Autodesk Inventor part; units mm, degrees
ref_plane "YZ Plane" through (0, 0, 0) normal (1, 0, 0) x (0, 1, 0)
ref_plane "XZ Plane" through (0, 0, 0) normal (0, 1, 0) x (-1, 0, 0)
ref_plane "XY Plane" through (0, 0, 0) normal (0, 0, 1) x (1, 0, 0)
sketch "Sketch1" plane through (0, 0, 0) normal (0, 0, 1) x (1, 0, 0)
  circle A0 centre (0, 0) radius 11
  circle A1 centre (-15.5, 15.5) radius 1.5
  circle A2 centre (15.5, 15.5) radius 1.5
  circle A3 centre (-15.5, -15.5) radius 1.5
  circle A4 centre (15.5, -15.5) radius 1.5
  line L0 (21.05, -21.05) -> (-21.05, -21.05)
  line L1 (21.05, 21.05) -> (21.05, -21.05)
  line L2 (-21.05, 21.05) -> (21.05, 21.05)
  line L3 (-21.05, -21.05) -> (-21.05, 21.05)
  point P0 (0, 0)
extrude "Extrusion1" add sketch "Sketch1" along normal blind 8
sketch "Sketch2" plane through (-21.05, 21.05, 0) normal (0, 1, 0) x (1, 0, 0)
  line L0 (42.1, 0) -> (0, 0)
  line L1 (0, 0) -> (0, -8)
  line L2 (42.1, -8) -> (0, -8)
  line L3 (42.1, 0) -> (42.1, -8)
  point P0 (21.05, 0)
extrude "Extrusion2" add sketch "Sketch2" along normal blind 50
properties part number "nema17 x plate"
Work out the finished part from the listing and answer in its coordinate system (mm). Round coordinates to 2 decimals unless told otherwise and drop trailing zeros. Write each loop counter-clockwise with the first axis right and the second up, starting at its lowest first coordinate (ties: lowest second). Pieces come first, ordered by that corner, then holes. Notation, with made-up numbers: (-13, -16.5) - (43, -16.5) arc R27 cw to (43, 0.5) - close; hole circle Ø2 at (-8, -3). An arc over 180 degrees is marked (long way). Return JSON: item names as keys, results as strings. Group by question number.
Q1. The part is cut by section C-C on y = 15.5. Write down the section's boundary in (x, z).
Q2. The mould has two halves that part along X. Classify faces 1 (the cylindrical face through (-17, 15.43, 3.94)), 2 (the flat face through (0, 71.05, 4)), 3 (the flat face through (21.05, 26, 4)), 4 (the cylindrical face through (-17, -15.57, 3.94)): released by +X, released by -X, zero draft, split by the parting line, or undercut.
Q3. The part is cut by section B-B on x = 0. Write down the section's boundary in (y, z), then the cut area to 3 significant figures.
Q4. The part is cut by section D-D on x = 15.5. Write down the section's boundary in (y, z).
Q5. Find the intervals of material crossed by L1, parallel to X at y = 14.5, z = 7.5; L2, parallel to Y at x = -15, z = 3.5; L3, parallel to Y at x = 2, z = 3.75, in increasing order.
Q6. The part is cut by section A-A on y = 0. Write down the section's boundary in (x, z).
Solved:
{
 "1": {"outline": "(-21.05, 0) - (-17, 0) - (-17, 8) - (-21.05, 8) - close; (-14, 0) - (14, 0) - (14, 8) - (-14, 8) - close; (17, 0) - (21.05, 0) - (21.05, 8) - (17, 8) - close"},
 "2": {"face 1": "undercut", "face 2": "zero draft", "face 3": "released by +X", "face 4": "undercut"},
 "3": {"outline": "(-21.05, 0) - (-11, 0) - (-11, 8) - (-21.05, 8) - close; (11, 0) - (71.05, 0) - (71.05, 8) - (11, 8) - close", "area": "561 mm²"},
 "4": {"outline": "(-21.05, 0) - (-17, 0) - (-17, 8) - (-21.05, 8) - close; (-14, 0) - (14, 0) - (14, 8) - (-14, 8) - close; (17, 0) - (71.05, 0) - (71.05, 8) - (17, 8) - close"},
 "5": {"L1": "-21.05 to -16.62, -14.38 to 14.38, 16.62 to 21.05", "L2": "-21.05 to -16.91, -14.09 to 14.09, 16.91 to 71.05", "L3": "-21.05 to -10.82, 10.82 to 71.05"},
 "6": {"outline": "(-21.05, 0) - (-11, 0) - (-11, 8) - (-21.05, 8) - close; (11, 0) - (21.05, 0) - (21.05, 8) - (11, 8) - close"}
}
